Could you check a few things on this drawing? It's one solid part, dimensions in mm from its lowest x, y, z. A direction names the side the tool comes from. Coordinates: 2 decimals unless noted, no trailing zeros. Write each loop counter-clockwise with the first axis right and the second up, starting at its lowest first coordinate (ties: lowest second). Pieces come first, ordered by that corner, then holes.
Item 1: I want a section at A-A (y = 40). Please give me the cut outline in (x, z).
Item 2: I want a section at C-C (x = 13.5). Please give me the cut outline in (y, z), and give its area (3 significant figures).
Item 3: I want a section at D-D (y = 13). Please give me the cut outline in (x, z) (1 decimal).
Item 4: I'm going to push a flat-ended pin straight in: P1, Ø16, axis at x = 22.21, y = 16.96, coming from the -Z side. Where does the tip first touch, or does it pass through?
Item 5: Please list where these lines run through material, in increasing order: line 1 (X direction, y = 40, z = 49); line 2 (Z direction, x = 8, y = 46); line 3 (Y direction, x = 50, z = 3).
Item 6: If we mould it in two halves opening along Y, with no side actions, what happens to the marked faces 1, 2 and 3? For each: pulls with the +Y half, pulls with the -Y half, needs draft (parallel to the pull), parting line crosses it, or undercut.
Item 7: For the marked faces 4, 5 and 6, which set-ups out of +Z, -Z, +X, -X, +Y, -Y let a thin tool reach every point of the face, with its end or its side?
Item 8: I want a section at B-B (x = 38.5). Please give me the cut outline in (y, z).
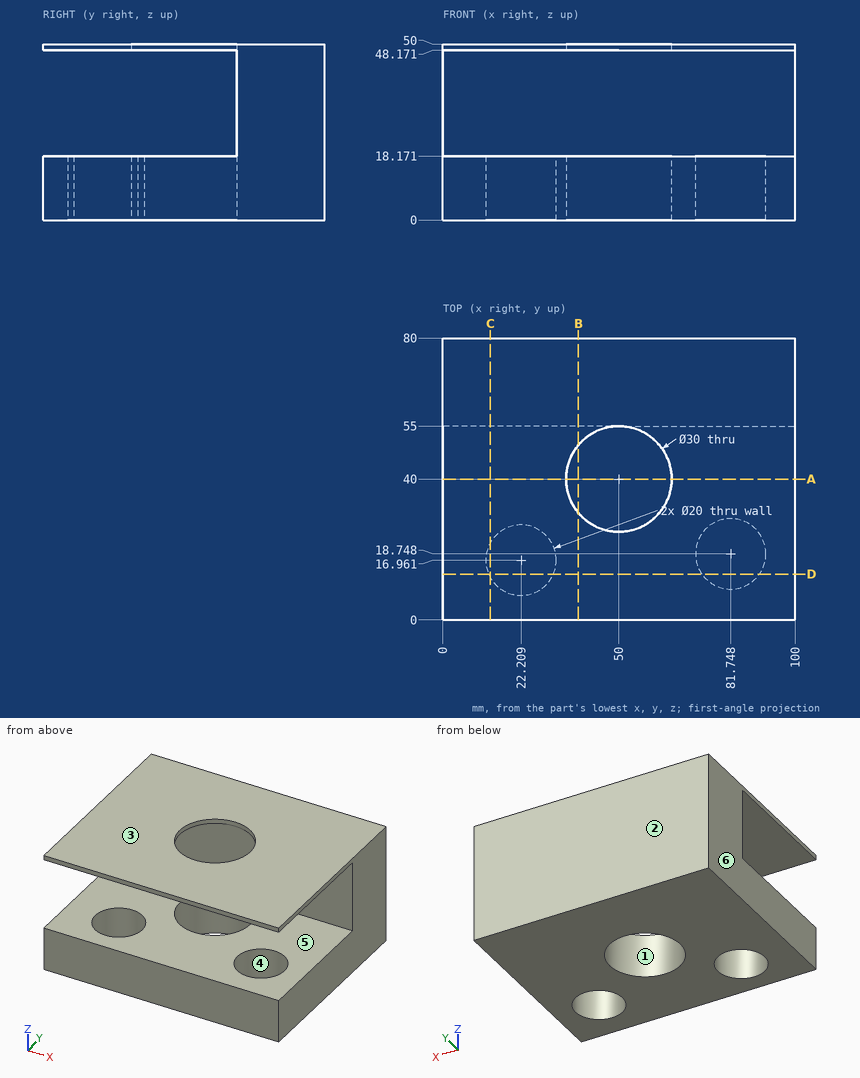
Answer:
1. outline: (0, 0) - (35, 0) - (35, 18.17) - (0, 18.17) - close; (0, 48.17) - (35, 48.17) - (35, 50) - (0, 50) - close; (65, 0) - (100, 0) - (100, 18.17) - (65, 18.17) - close; (65, 48.17) - (100, 48.17) - (100, 50) - (65, 50) - close
2. outline: (0, 0) - (12.05, 0) - (12.05, 18.17) - (0, 18.17) - close; (0, 48.17) - (55, 48.17) - (55, 18.17) - (21.88, 18.17) - (21.88, 0) - (80, 0) - (80, 50) - (0, 50) - close
2. area: 2,170 mm2
3. outline: (0, 0) - (13, 0) - (13, 18.2) - (0, 18.2) - close; (0, 48.2) - (100, 48.2) - (100, 50) - (0, 50) - close; (31.4, 0) - (73.6, 0) - (73.6, 18.2) - (31.4, 18.2) - close; (89.9, 0) - (100, 0) - (100, 18.2) - (89.9, 18.2) - close
4. P1: stops at z = 48.17
5. line 1: x = 0 to 35, 65 to 100
5. line 2: z = 0 to 18.17, 48.17 to 50
5. line 3: y = 0 to 25, 55 to 80
6. face 1: undercut
6. face 2: pulls with the +Y half
6. face 3: needs draft
7. face 4: -Z
7. face 5: +X, -X, -Y
7. face 6: +Z, -Z, -X, +Y, -Y
8. outline: (0, 0) - (30.37, 0) - (30.37, 18.17) - (0, 18.17) - close; (0, 48.17) - (30.37, 48.17) - (30.37, 50) - (0, 50) - close; (49.63, 0) - (80, 0) - (80, 50) - (49.63, 50) - (49.63, 48.17) - (55, 48.17) - (55, 18.17) - (49.63, 18.17) - close
